Autodesk Inventor part; units mm, degrees
ref_plane "YZ Plane" through (0, 0, 0) normal (1, 0, 0) x (0, 1, 0)
ref_plane "XZ Plane" through (0, 0, 0) normal (0, 1, 0) x (-1, 0, 0)
ref_plane "XY Plane" through (0, 0, 0) normal (0, 0, 1) x (1, 0, 0)
sketch "Sketch1" plane through (0, 0, 0) normal (0, 0, 1) x (1, 0, 0)
  line L0 (0, 0) -> (37, 0)
  line L1 (37, 0) -> (39.3087, 10)
  line L2 (39.3087, 10) -> (0, 10)
  line L3 (0, 10) -> (0, 0)
  dimension "d0" = 77
  dimension "d2" = 37
  dimension "d3" = 10
revolve "Revolution1" add sketch "Sketch1" angle 360 about axis through (0, 10, 0) along (0, -1, 0)
shell "Shell1" thickness 1.2 removed faces 1 at (-11.8053, 10, 5.6851)
fillet "Fillet1" radius 1 1 edges at (-36.0455, 1.2, 0)
sketch "Sketch2" plane through (0, 0, 0) normal (0, -1, 0) x (1, 0, 0)
  circle A0 centre (0, 0) radius 37
  arc A1 (9.3175, 34.7733) -> (-9.3175, 34.7733) centre (0, 0) ccw
  line L0 (-9.3175, 34.7733) -> (-9.5763, 35.7393)
  line L1 (0, 0) -> (0, 37)
  line L2 (9.3175, 34.7733) -> (9.5763, 35.7393)
  arc A2 (9.5763, 35.7393) -> (-9.5763, 35.7393) centre (0, 0) ccw
  point P0 (0, 0)
  dimension "d8" = 72
  dimension "d9" = 15
  dimension "d10" = 15
extrude "Extrusion1" add sketch "Sketch2" along normal blind 1.5 contours L2 A1 L1 A0 | A0 L1 A1 L0
pattern_circular "Circular Pattern1" count 6 over 360 about axis through (0, -10, 0) along (0, 1, 0) of "Extrusion1"
properties part number "pot_holder_prototype"
Design review of the part built by this model. Coordinates are the model's own, in mm. A direction names the side the tool comes from. Coordinates: 2 decimals unless noted, no trailing zeros. Order: outer loops, then holes, each group sorted by start corner. A loop starts at its lowest first (then second) coordinate and runs counter-clockwise, first axis right, second up. Notation, with made-up numbers: (32, -13.75) - (91, -13.75) arc R24 cw to (91, 10.25) - close; hole circle Ø9 at (47, 66.25). An arc over 180 degrees is marked (long way). Put each result on its own line as item: value.
1) Take a section at A-A, the plane z = 0. Give the boundary of the cut face in (x, y).
Response values:
outline: (-39.31, 10) - (-37, 0) - (37, 0) - (39.31, 10) - (38.08, 10) - (36.22, 1.98) arc R1 cw to (35.25, 1.2) - (-35.25, 1.2) arc R1 cw to (-36.22, 1.98) - (-38.08, 10) - close
2) Wall thickness on L1, parallel to X at y = 3, z = 24.5; L2, parallel to Y at x = -4, z = -2; L3, parallel to Z at x = 6, y = 3.5: over which ranges is each line inside the solid? List them lowest first. Write a range as from..to.
Response values:
L1: x = -28.64..-27, 27..28.64
L2: y = 0..1.2
L3: z = -37.33..-36.08, 36.08..37.33
3) Take a section at B-B, the plane x = 0. Give the boundary of the cut face in (y, z), and give its area (3 significant figures).
Response values:
outline: (-1.5, -37) - (0, -37) - (10, -39.31) - (10, -38.08) - (1.98, -36.22) arc R1 cw to (1.2, -35.25) - (1.2, 35.25) arc R1 cw to (1.98, 36.22) - (10, 38.08) - (10, 39.31) - (0, 37) - (-1.5, 37) - (-1.5, 36) - (0, 36) - (0, -36) - (-1.5, -36) - close
area: 114 mm²
4) The part is to be moulded in two halves that separate along X. For faces 1 (the face through (-8.052, 0.626, 36.261)), 2 (the face through (-31.5, -1.5, -18.3)), 3 (the face through (-31.975, -0.74, -18.617)), 4 (the face through (-31.24, -0.74, 17.89)), say which applies: released by +X, released by -X, zero draft, split by the parting line, or undercut.
Response values:
face 1: split by the parting line
face 2: zero draft
face 3: released by -X
face 4: undercut
5) Take a section at C-C, the plane y = 6.75. Give the boundary of the cut face in (x, z), and give its area (3 significant figures).
Response values:
outline: circle Ø77.12 at (0, 0); hole circle Ø74.65 at (0, 0)
area: 294 mm²
6) Tool access review of faces 5 (the face through (-1, 0, 1)), 6 (the face through (-0.13, -1.5, 36.15)), 7 (the face through (-32.1, -0.7, 18.4)), 8 (the face through (31.975, -0.74, 18.617)), 9 (the face through (32.1, -0.7, -18.4)): name each direction out of +Z, -Z, +X, -X, +Y, -Y from which nothing blocks a thin tool from reaching the whole face with its end or side.
Response values:
face 5: -Y
face 6: +Z, -Z, +X, -X, -Y
face 7: +Z, -X, -Y
face 8: +Z, +X, -Y
face 9: -Z, +X, -Y
7) Insertion check: P1, Ø3, axis at x = 10.5, z = -28, coming from the +Y side; P2, Ø1.5, axis at x = -23.5, y = 3.5, coming from the +Z side; P3, Ø5, axis at y = 1, z = -27, coming from the -X side. Each pin has a flat end and moves straight along its axis. Give the tip position at first contact, or say it passes through.
Response values:
P1: stops at y = 1.2
P2: stops at z = 30.24
P3: stops at x = -28.16
